Could you check a few things on this model? Use its own coordinates, in mm. A direction names the side the tool comes from. Round coordinates to 2 decimals unless told otherwise and drop trailing zeros. Loops run counter-clockwise (first coordinate to the right, second up) from the corner with the lowest first, then second, coordinate; pieces in that order, holes last. Notation, with made-up numbers: M 84.5,48 L 138.5,48 A28 ccw 138.5,70 Z; hole C -39,21.25 d1. An arc over 180 degrees is marked long. Answer in a Markdown table with one row per item.
```python
from build123d import *

# Parameters (mm, degrees)
SKETCH_W     = 34.16
SKETCH_H     = 18.62
PAD_DEPTH    = 2.6
SKETCH002_R  = 0.5
SKETCH002_W  = 24.92
SKETCH002_H  = 12.92
POCKET_DEPTH = 2.6


with BuildPart() as part:
    # Sketch → Pad (new body)
    with BuildSketch(Plane.XZ):
        with Locations((17.08, 9.31)):
            Rectangle(SKETCH_W, SKETCH_H)
    extrude(amount=PAD_DEPTH)

    # Sketch002 (on Face6 of Pad) → Pocket (cut)
    with BuildSketch(Plane.XZ.offset(2.6)):
        with Locations((2.31, 1.425)):
            Circle(SKETCH002_R)
        with Locations((17.08, 9.31)):
            Rectangle(SKETCH002_W, SKETCH002_H)
    extrude(amount=-POCKET_DEPTH, mode=Mode.SUBTRACT)


solid = part.part
```
1) I want a section at B-B, the plane z = 13.25. Please give me the cut outline in (x, y), plus the area to 3 significant figures.
Computed:
| item | result |
|---|---|
| outline | M 0,-2.6 L 4.62,-2.6 L 4.62,0 L 0,0 Z; M 29.54,-2.6 L 34.16,-2.6 L 34.16,0 L 29.54,0 Z |
| area | 24.0 mm² |
2) I want a section at A-A, the plane x = 2.31. Please give me the cut outline in (y, z) (3 decimals), plus the area to 3 significant figures.
Computed:
| item | result |
|---|---|
| outline | M -2.6,0 L 0,0 L 0,0.925 L -2.6,0.925 Z; M -2.6,1.925 L 0,1.925 L 0,18.62 L -2.6,18.62 Z |
| area | 45.8 mm² |
3) If we mould it in two halves opening along Z, with no side actions, what happens to faces 3 (the face through (1.81, -1.32, 1.45)), 4 (the face through (17, 0, 18)), 5 (the face through (17, -1, 0)), 6 (the face through (29.54, -1, 9))? For each: released by +Z, released by -Z, zero draft, split by the parting line, or undercut.
Computed:
| item | result |
|---|---|
| face 3 | undercut |
| face 4 | zero draft |
| face 5 | released by -Z |
| face 6 | undercut |
4) I want a section at C-C, the plane y = -1.15. Please give me the cut outline in (x, z) (3 decimals), plus the area to 3 significant figures.
Computed:
| item | result |
|---|---|
| outline | M 0,0 L 34.16,0 L 34.16,18.62 L 0,18.62 Z; hole C 2.31,1.425 d1; hole M 4.62,2.85 L 29.54,2.85 L 29.54,15.77 L 4.62,15.77 Z |
| area | 313 mm² |
5) Which directions (+Z, -Z, +X, -X, +Y, -Y) give clear straight access to the entire face, cutting with the end or side of a thin tool? Please do faces 1 (the face through (0, -1, 9)), 2 (the face through (4.62, -1, 9)).
Computed:
| item | result |
|---|---|
| face 1 | +Z, -Z, -X, +Y, -Y |
| face 2 | +Y, -Y |
6) I need wall thicknesses on line 1 (X direction, y = -1.15, z = 11.75); line 2 (Z direction, x = 6, y = -0.6); line 3 (Z direction, x = 2.31, y = -1.65) (3 decimals). Which ranges of each line are inside material? Lowest first, please.
Computed:
| item | result |
|---|---|
| line 1 | x = 0 to 4.62, 29.54 to 34.16 |
| line 2 | z = 0 to 2.85, 15.77 to 18.62 |
| line 3 | z = 0 to 0.925, 1.925 to 18.62 |
